The model under review builds one solid part; all positions refer to its coordinate system, in mm. Face numbers are marked on the shaded views. A direction names the side the tool comes from. Coordinates: 2 decimals unless noted, no trailing zeros. Write each loop counter-clockwise with the first axis right and the second up, starting at its lowest first coordinate (ties: lowest second). Pieces come first, ordered by that corner, then holes. Notation, with made-up numbers: M -39,21 L 10,21 A20 ccw 10,38 Z; hole C 79.5,57 d7. An arc over 180 degrees is marked long. Answer as CSV lines item,"result". Start each with the question number.
from build123d import *

# Parameters (mm, degrees)
F0_W     = 107
F0_H     = 102
F1_DEPTH = 40
F2_W     = 38
F2_H     = 102
F2_W_2   = 28
F3_DEPTH = 30
F5_D     = 8
F5_DEPTH = 20
F5_TIP   = 2.4034424761
F7_D     = 5
F9_D     = 12


with BuildPart() as f1:
    # F0 (on Top) → F1 (new body)
    with BuildSketch(Plane.XY):
        Rectangle(F0_W, F0_H)
    extrude(amount=F1_DEPTH)

    # F2 (on face) → F3 (cut)
    with BuildSketch(Plane.XY.offset(40)):
        with Locations((-34.5, 0)):
            Rectangle(F2_W, F2_H)
        with Locations((39.5, 0)):
            Rectangle(F2_W_2, F2_H)
    extrude(amount=-F3_DEPTH, mode=Mode.SUBTRACT)

    # F5
    with Locations(Plane(origin=(0, 0, 0), x_dir=(1, 0, 0), z_dir=(0, 0, -1))):
        with Locations((-5, -18), (-5, -36), (15, -36), (15, -18), (-5, 0), (15, 0), (15, 18), (-5, 18), (-5, 36), (15, 36)):
            Hole(F5_D / 2, depth=F5_DEPTH)
            with Locations((0, 0, -(F5_DEPTH + F5_TIP / 2))):  # 118° drill point
                Cone(0, F5_D / 2, F5_TIP, mode=Mode.SUBTRACT)

    # F7 (through all)
    with Locations(Plane.XY.offset(40)):
        with Locations((-5, -36), (15, -36), (-5, -18), (15, -18), (-5, 0), (15, 0), (-5, 18), (15, 18), (-5, 36), (15, 36)):
            Hole(F7_D / 2)

    # F9 (through all)
    with Locations(Plane(origin=(0, 0, 0), x_dir=(1, 0, 0), z_dir=(0, 0, -1))):
        with Locations((-40, 26), (-40, -26), (40, -26), (40, 26)):
            Hole(F9_D / 2)


solid = f1.part
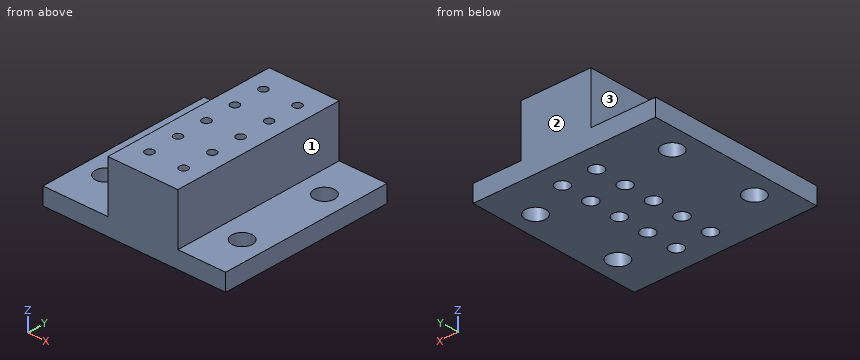
1) To check wall thickness, follow line 1 (Y direction, x = 15, z = 36); line 2 (X direction, y = -36, z = 4); line 3 (X direction, y = 18, z = 35). State the ranges of each line that lie inside material, in increasing order. Write a range as [from, to].
2) Tool access review of the marked faces 1, 2 and 3: name each direction out of +Z, -Z, +X, -X, +Y, -Y from which nothing blocks a thin tool from reaching the whole face with its end or side.
3) Take a section at A-A on x = 40. Give the boundary of the cut face in (y, z).
4) Clearance check with flat-ended pins moving along their axes: pin 1 Ø9.5 at (x, y) = (-40, 26) entering from -Z; pin 2 Ø8 at (y, z) = (5, 23) entering from -X; pin 3 Ø7 at (x, y) = (15, -18) entering from -Z; pin 4 Ø14 at (x, y) = (40, 26) entering from +Z. State where each tip first meets the part, or that it passes through.
5) Take a section at C-C on z = 16.5. Give the number of separate pieces and of enclosed holes in the cut face, and give its area (3 significant figures).
6) Take a section at B-B on y = -36. Give the boundary of the cut face in (x, z), and give its area (3 significant figures).
Results:
1,line 1,"y = [-51, -38.5], [-33.5, -20.5], [-15.5, -2.5], [2.5, 15.5], [20.5, 33.5], [38.5, 51]"
1,line 2,"x = [-53.5, -9], [-1, 11], [19, 53.5]"
1,line 3,"x = [-15.5, -7.5], [-2.5, 12.5], [17.5, 25.5]"
2,face 1,"+Z, +X, +Y, -Y"
2,face 2,"+Z, -Z, +X, -X, +Y"
2,face 3,"+Z, -X, +Y, -Y"
3,outline,"M -51,0 L -32,0 L -32,10 L -51,10 Z; M -20,0 L 20,0 L 20,10 L -20,10 Z; M 32,0 L 51,0 L 51,10 L 32,10 Z"
4,pin 1,"passes through"
4,pin 2,"stops at x = -15.5"
4,pin 3,"stops at z = 20.3"
4,pin 4,"stops at z = 10"
5,separate pieces,"1"
5,enclosed holes,"10"
5,area,"3,680 mm²"
6,outline,"M -53.5,0 L -9,0 L -9,20 L -7.5,20.9 L -7.5,40 L -15.5,40 L -15.5,10 L -53.5,10 Z; M -2.5,20.9 L -1,20 L -1,0 L 11,0 L 11,20 L 12.5,20.9 L 12.5,40 L -2.5,40 Z; M 17.5,20.9 L 19,20 L 19,0 L 53.5,0 L 53.5,10 L 25.5,10 L 25.5,40 L 17.5,40 Z"
6,area,"1,780 mm²"
